```python
from build123d import *

# Parameters (mm, degrees)
F0_R      = 26.0164599328
F1_DEPTH  = 108.204
F2_W      = 50.4153975605
F2_H      = 92.5804451108
F3_DEPTH  = 13.97
F4_W      = 50.4153975605
F4_H      = 99.2666035891
F5_DEPTH  = 16.002
F6_W      = 16.002
F6_H      = 7.0882067084
F7_DEPTH  = 64.008
F8_R      = 12.9022316947
F9_DEPTH  = 152.146
F11_DEPTH = 15.748
F13_DEPTH = 13.97
F14_R     = 13.5333252063
F15_DEPTH = 238.252


with BuildPart() as f1:
    # F0 (on Front) → F1 (new body)
    with BuildSketch(Plane.XZ):
        with Locations((-32.4612818658, 6.4364671707)):
            Circle(F0_R)
    extrude(amount=F1_DEPTH)

    # F2 (on face) → F3 (join)
    with BuildSketch(Plane.XZ.offset(108.204)):
        with Locations((-32.4612818658, 46.2902225554)):
            Rectangle(F2_W, F2_H)
    extrude(amount=-F3_DEPTH)

    # F4 (on face) → F5 (join)
    with BuildSketch(Plane(origin=(0, 0, 0), x_dir=(-1, 0, 0), z_dir=(0, 1, 0))):
        with Locations((32.4612818658, 49.6333017945)):
            Rectangle(F4_W, F4_H)
    extrude(amount=-F5_DEPTH)

    # F6 (on face) → F7 (cut)
    with BuildSketch(Plane.YZ.offset(-7.2535830856)):
        with Locations((-8.001, 95.7225002348)):
            Rectangle(F6_W, F6_H)
    extrude(amount=-F7_DEPTH, mode=Mode.SUBTRACT)

    # F8 (on face) → F9 (cut)
    with BuildSketch(Plane.XZ.offset(108.204)):
        with Locations((-32.4612818658, 6.4364671707)):
            Circle(F8_R)
    extrude(amount=-F9_DEPTH, mode=Mode.SUBTRACT)

    # F10 (on face) → F11 (join)
    with BuildSketch(Plane(origin=(0, 0, 0), x_dir=(-1, 0, 0), z_dir=(0, 1, 0))):
        with BuildLine():
            Line((7.2535830856, 92.1783968806), (57.6689806461, 92.1783968806))
            ThreePointArc((57.6689806461, 92.1783968806), (32.4612818658, 117.3860956609), (7.2535830856, 92.1783968806))
        make_face()
    extrude(amount=-F11_DEPTH)

    # F12 (on face) → F13 (join)
    with BuildSketch(Plane.XZ.offset(108.204)):
        with BuildLine():
            Line((-57.6689806461, 92.5804451108), (-7.2535830856, 92.5804451108))
            ThreePointArc((-7.2535830856, 92.5804451108), (-32.4612818658, 117.7881438911), (-57.6689806461, 92.5804451108))
        make_face()
    extrude(amount=-F13_DEPTH)

    # F14 (on face) → F15 (cut)
    with BuildSketch(Plane.XZ.offset(108.204)):
        with Locations((-32.4612818658, 92.5804451108)):
            Circle(F14_R)
    extrude(amount=-F15_DEPTH, mode=Mode.SUBTRACT)


solid = f1.part
```
Check sheet for the modelled part. Datum: model origin and axes. Units: mm. A direction names the side the tool comes from. Coordinates: 2 decimals unless noted, no trailing zeros. Order: outer loops, then holes, each group sorted by start corner. A loop starts at its lowest first (then second) coordinate and runs counter-clockwise, first axis right, second up. Notation, with made-up numbers: M 75,-35 L 79,-35 A18 ccw 79,-5 Z; hole C -5.5,59 d5. An arc over 180 degrees is marked long. Write each question's results on one line, items separated by ' | '. Start each with the question number.
1. Cross-section at B-B on x = -24.5. Record the cut outline in (y, z).
2. Cross-section at C-C on x = -51. Record the cut outline in (y, z).
3. Mould release check, pull along Z, two halves, no side actions. Record for faces 6 (the face through (-42.7, -54.859, -1.414)), 7 (the face through (-33.02, -7.76, 117.38)), 8 (the face through (-32, 0, 50)): +Z half, -Z half, draft (parallel to the pull), parting line (faces both ways), or undercut.
4. Cross-section at A-A on z = 40.5. Record the cut outline in (x, y).
5. Cross-section at D-D on z = 11. Record the cut outline in (x, y).
6. Material ranges on probe 1 along Y at (x, z) = (-50, 54); probe 2 along Y at (x, z) = (-13.5, 105); probe 3 along Z at (x, y) = (-32, -46.5), recorded low to high.
7. Go/stop test with flat-tipped pins: P1, Ø13, axis at y = -5.5, z = 54.5, coming from the -X side; P2, Ø1, axis at x = -40.5, y = -30, coming from the +Z side; P3, Ø1.5, axis at y = -69.5, z = 4, coming from the +X side. Record where each tip stops, or that it passes through.
8. Access from +Z, -Z, +X, -X, +Y, -Y to the whole of each face (thin tool, end or side, straight path). Record for faces 1 (the face through (-25.2, -8.1, 104)), 2 (the face through (-7.254, -8, 52)), 3 (the face through (-32, -15.748, 108)), 4 (the face through (-57.669, -101, 52)), 5 (the face through (-38.1, -53.34, -18.96)).
Checks:
1) outline: M -108.2,-18.33 L 0,-18.33 L 0,-3.72 L -108.2,-3.72 Z; M -108.2,16.59 L 0,16.59 L 0,81.64 L -16,81.64 L -16,31.2 L -94.23,31.2 L -94.23,81.64 L -108.2,81.64 Z; M -108.2,103.52 L -94.23,103.52 L -94.23,116.5 L -108.2,116.5 Z; M -15.75,103.52 L 0,103.52 L 0,116.1 L -15.75,116.1 Z
2) outline: M -108.2,-11.82 L 0,-11.82 L 0,109.26 L -15.75,109.26 L -15.75,92.18 L -16,92.18 L -16,24.69 L -94.23,24.69 L -94.23,109.66 L -108.2,109.66 Z
3) face 6: undercut | face 7: +Z half | face 8: draft
4) outline: M -57.67,-108.2 L -7.25,-108.2 L -7.25,-94.23 L -57.67,-94.23 Z; M -57.67,-16 L -7.25,-16 L -7.25,0 L -57.67,0 Z
5) outline: M -58.07,-108.2 L -44.53,-108.2 L -44.53,0 L -58.07,0 Z; M -20.39,-108.2 L -6.85,-108.2 L -6.85,0 L -20.39,0 Z
6) probe 1: y = -108.2 to -94.23, -16 to 0 | probe 2: y = -108.2 to -94.23, -15.75 to 0 | probe 3: z = -19.58 to -6.46, 19.33 to 32.45
7) P1: stops at x = -57.67 | P2: stops at z = 31.34 | P3: stops at x = -6.5
8) face 1: +Y, -Y | face 2: +Z, +X, +Y, -Y | face 3: +Z, +X, -X | face 4: +Z, -X, +Y, -Y | face 5: none
